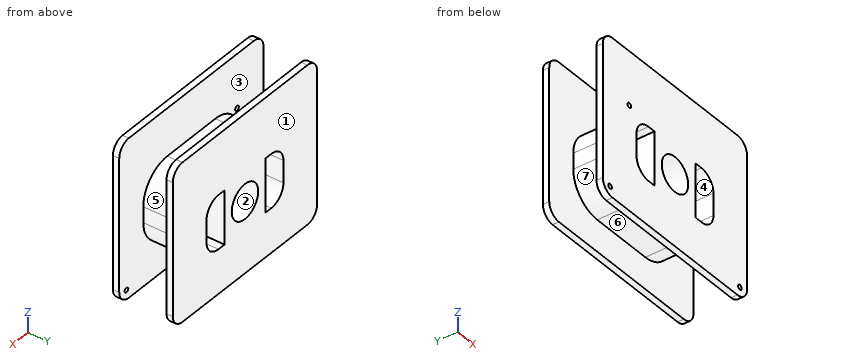
```python
from build123d import *

# Parameters (mm, degrees)
F0_W      = 60
F0_H      = 50
F0_R      = 5.5
F1_DEPTH  = 2
F2_W      = 40
F2_H      = 25
F2_R      = 5.5
F3_DEPTH  = 15
F4_R      = 10
F5_W      = 60
F5_H      = 50
F5_R      = 5.5
F6_DEPTH  = 2
F7_R      = 4
F9_D      = 1.5
F9_DEPTH  = 3
F9_TIP    = 0.4506454643
F10_W     = 7.5
F10_H     = 17
F11_DEPTH = 25
F12_R     = 5


# Not quite as in the source:
# - a feature names something its author has since deleted; it is built from what else it names


with BuildPart() as f1:
    # F0 (on Front) → F1 (new body)
    with BuildSketch(Plane.XZ):
        with Locations((0, 2.5)):
            Rectangle(F0_W, F0_H)
        Circle(F0_R, mode=Mode.SUBTRACT)
    extrude(amount=F1_DEPTH)

    # F2 (on face) → F3 (join)
    with BuildSketch(Plane.XZ.offset(2)):
        Rectangle(F2_W, F2_H)
        Circle(F2_R, mode=Mode.SUBTRACT)
    extrude(amount=F3_DEPTH)

    # F4
    f4_edges = [f1.edges().sort_by_distance(p)[0] for p in [
        (20, -9.5, 12.5),
        (20, -9.5, -12.5),
        (-20, -9.5, -12.5),
        (-20, -9.5, 12.5),
    ]]
    fillet(f4_edges, radius=F4_R)

    # F5 (on face) → F6 (join)
    with BuildSketch(Plane.XZ.offset(17)):
        with Locations((0, 2.5)):
            Rectangle(F5_W, F5_H)
        Circle(F5_R, mode=Mode.SUBTRACT)
    extrude(amount=F6_DEPTH)

    # F7
    f7_edges = [f1.edges().sort_by_distance(p)[0] for p in [
        (30, -18, 27.5),
        (30, -1, 27.5),
        (30, -18, -22.5),
        (30, -1, -22.5),
        (-30, -18, -22.5),
        (-30, -1, -22.5),
        (-30, -18, 27.5),
        (-30, -1, 27.5),
    ]]
    fillet(f7_edges, radius=F7_R)

    # F9
    with Locations(Plane.XZ.offset(19)):
        with Locations((-19, 10.5), (-27, -19.5), (27, -19.5)):
            Hole(F9_D / 2, depth=F9_DEPTH)
            with Locations((0, 0, -(F9_DEPTH + F9_TIP / 2))):  # 118° drill point
                Cone(0, F9_D / 2, F9_TIP, mode=Mode.SUBTRACT)

    # F10 (on face) → F11 (cut)
    with BuildSketch(Plane.XZ.offset(19)):
        with Locations((-12.25, 0)):
            Rectangle(F10_W, F10_H)
        with Locations((12.25, 0)):
            Rectangle(F10_W, F10_H)
    extrude(amount=-F11_DEPTH, mode=Mode.SUBTRACT)

    # F12
    f12_edges = [f1.edges().sort_by_distance(p)[0] for p in [
        (16, -9.5, -8.5),
        (16, -9.5, 8.5),
        (-16, -9.5, 8.5),
        (-16, -9.5, -8.5),
    ]]
    fillet(f12_edges, radius=F12_R)


solid = f1.part
```
Design review of the part built by this model. Coordinates are the model's own, in mm. Face numbers are marked on the shaded views. A direction names the side the tool comes from. Give positions to 0.01 mm unless a question says otherwise; leave off trailing zeros. Write each loop counter-clockwise with the first axis right and the second up, starting at its lowest first coordinate (ties: lowest second). Pieces come first, ordered by that corner, then holes. Notation, with made-up numbers: (17, 0) - (30, 0) arc R11 cw to (30, 13) - close; hole circle Ø9 at (-18.5, 3.25). An arc over 180 degrees is marked (long way). Return JSON: item names as keys, results as strings. Group by question number.
(1) We need section A-A, the plane x = -23. Give the boundary of the cut face in (y, z).
(2) We need section D-D, the plane z = 0. Give the boundary of the cut face in (x, y).
(3) We need section B-B, the plane z = 10.5. Give the boundary of the cut face in (x, y).
(4) To check wall thickness, follow probe 1 along Y at (x, z) = (-24.5, 19.5); probe 2 along Z at (x, y) = (-19, -18.45); probe 3 along X at (y, z) = (-11, 0.5). State the ranges of each line that lie inside material, in increasing order.
(5) We need section C-C, the plane y = -9.5. Give the boundary of the cut face in (x, z), then the cut area to 3 significant figures.
(6) Mouldability with a two-part tool opening along Y and no side actions: class the marked faces 1, 2 and 3 as +Y half, -Y half, draft (parallel to the pull), parting line (faces both ways), or undercut.
(7) Insertion check: pin 1 (5 mm diameter, centred on y = -14, z = 3.5, fed in from -X); pin 2 (0.9 mm diameter, centred on x = -19, z = 10.5, fed in from -Y); pin 3 (2 mm diameter, centred on x = 22, y = -5, fed in from +Z); pin 4 (2 mm diameter, centred on x = -10, y = -6, fed in from +Z). Each pin has a flat end and moves straight along its axis. Give the tip position at first contact, or say it passes through.
(8) Machinability: for the marked faces 4, 5, 6 and 7, which of the approach directions +Z, -Z, +X, -X, +Y, -Y give a long, thin tool a straight path to every point of the face, cutting with its end or side? Answer none if there is none.
Reported:
{
 "1": {"outline": "(-19, -22.5) - (-17, -22.5) - (-17, 27.5) - (-19, 27.5) - close; (-2, -22.5) - (0, -22.5) - (0, 27.5) - (-2, 27.5) - close"},
 "2": {"outline": "(-30, -19) - (-16, -19) - (-16, 0) - (-30, 0) - (-30, -2) - (-20, -2) - (-20, -17) - (-30, -17) - close; (-8.5, -19) - (-5.5, -19) - (-5.5, 0) - (-8.5, 0) - close; (5.5, -19) - (8.5, -19) - (8.5, 0) - (5.5, 0) - close; (16, -19) - (30, -19) - (30, -17) - (20, -17) - (20, -2) - (30, -2) - (30, 0) - (16, 0) - close"},
 "3": {"outline": "(-30, -19) - (-19.75, -19) - (-19.75, -17) - (-30, -17) - close; (-30, -2) - (-16, -2) - (-16, -17) - (-18.25, -17) - (-18.25, -19) - (30, -19) - (30, -17) - (16, -17) - (16, -2) - (30, -2) - (30, 0) - (-30, 0) - close"},
 "4": {"probe 1": "y = -19 to -17, -2 to 0", "probe 2": "z = -22.5 to 9.75, 11.25 to 27.5", "probe 3": "x = -20 to -16, -8.5 to -5.48, 5.48 to 8.5, 16 to 20"},
 "5": {"outline": "(-20, -2.5) arc R10 ccw to (-10, -12.5) - (10, -12.5) arc R10 ccw to (20, -2.5) - (20, 2.5) arc R10 ccw to (10, 12.5) - (-10, 12.5) arc R10 ccw to (-20, 2.5) - close; hole (-16, -3.5) arc R5 ccw to (-11, -8.5) - (-8.5, -8.5) - (-8.5, 8.5) - (-11, 8.5) arc R5 ccw to (-16, 3.5) - close; hole circle Ø11 at (0, 0); hole (8.5, -8.5) - (11, -8.5) arc R5 ccw to (16, -3.5) - (16, 3.5) arc R5 ccw to (11, 8.5) - (8.5, 8.5) - close", "area": "586 mm2"},
 "6": {"face 1": "+Y half", "face 2": "draft", "face 3": "undercut"},
 "7": {"pin 1": "stops at x = -20", "pin 2": "stops at y = -2", "pin 3": "passes through", "pin 4": "stops at z = 12.5"},
 "8": {"face 4": "+Y, -Y", "face 5": "+Z, +X", "face 6": "-Z, +X, -X", "face 7": "-Z, -X"}
}
